Verification items for the finished model (mm, model axes). Face numbers are marked on the shaded views. A direction names the side the tool comes from. Round coordinates to 2 decimals unless told otherwise and drop trailing zeros. Write each loop counter-clockwise with the first axis right and the second up, starting at its lowest first coordinate (ties: lowest second). Pieces come first, ordered by that corner, then holes. Notation, with made-up numbers: (-35, -27) -> (18, -27) arc R24 ccw to (18, -10) -> close; hole circle Ø11 at (83, -1). An arc over 180 degrees is marked (long way). Use CSV: the item, a comma, the result in double quotes.
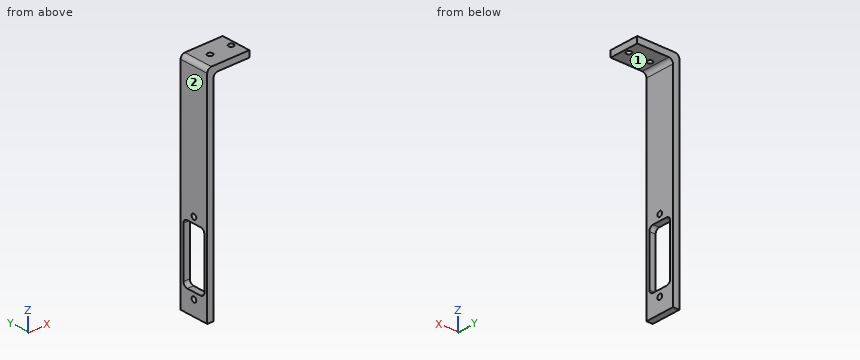
Autodesk Inventor part; units mm, degrees
ref_plane "YZ Plane" through (0, 0, 0) normal (1, 0, 0) x (0, 1, 0)
ref_plane "XZ Plane" through (0, 0, 0) normal (0, 1, 0) x (-1, 0, 0)
ref_plane "XY Plane" through (0, 0, 0) normal (0, 0, 1) x (1, 0, 0)
sketch "Sketch1" plane through (0, 0, 0) normal (0, 1, 0) x (-1, 0, 0)
  line L0 (0, 0) -> (0, -3)
  line L1 (0, -3) -> (15, -3)
  line L2 (17, -5) -> (17, -102.86)
  line L3 (0, 0) -> (18, 0)
  line L4 (20, -2) -> (20, -102.86)
  line L5 (20, -102.86) -> (17, -102.86)
  arc A0 (17, -5) -> (15, -3) centre (15, -5) ccw
  arc A1 (20, -2) -> (18, 0) centre (18, -2) ccw
  point P0 (17, -3)
  point P1 (20, 0)
  dimension "d0" = 3
  dimension "d1" = 17
  dimension "d2" = 99.86
  dimension "d3" = 20
  dimension "d4" = 2
extrude "Extrusion1" add sketch "Sketch1" along normal blind 14
sketch "Sketch2" plane through (0, 0, -3) normal (0, 0, -1) x (-1, 0, 0)
  point P0 (0, 0)
sketch "Sketch3" plane through (0, 0, -3) normal (0, 0, -1) x (-1, 0, 0)
  circle A0 centre (2.3646, 7) radius 1.5
  circle A1 centre (12.3646, 7) radius 1.5
  line L0 (0, 14) -> (15, 14)
  line L1 (0, 0) -> (15, 0)
  dimension "d7" = 3
  dimension "d8" = 3
  dimension "d9" = 14
  dimension "d10" = 7
  dimension "d11" = 10
hole "Hole1" at (-2.3646, 7, -3) at (-12.3646, 7, -3) direction (0, 0, 1) diameter 2.459 depth 8.8 tip angle 118
sketch "Sketch4" plane through (-20, 0, -102.86) normal (-1, 0, 0) x (0, 0, 1)
  line L0 (12, 12.5) -> (35.5, 12.5)
  line L1 (37.5, 10.5) -> (37.5, 3.5)
  line L2 (35.5, 1.5) -> (12, 1.5)
  line L3 (10, 3.5) -> (10, 10.5)
  line L4 (0, 14) -> (100.86, 14)
  line L5 (0, 0) -> (100.86, 0)
  line L6 (0, 0) -> (0, 14)
  circle A0 centre (7, 7) radius 1.5
  circle A1 centre (40.32, 7) radius 1.5
  arc A2 (12, 12.5) -> (10, 10.5) centre (12, 10.5) ccw
  arc A3 (10, 3.5) -> (12, 1.5) centre (12, 3.5) ccw
  arc A4 (37.5, 10.5) -> (35.5, 12.5) centre (35.5, 10.5) ccw
  arc A5 (35.5, 1.5) -> (37.5, 3.5) centre (35.5, 3.5) ccw
  point P0 (102.86, 0)
  point P1 (10, 12.5)
  point P2 (37.5, 1.5)
  point P3 (37.5, 12.5)
  point P4 (10, 1.5)
  dimension "d19" = 27.5
  dimension "d20" = 11
  dimension "d21" = 14
  dimension "d22" = 1.5
  dimension "d23" = 10
  dimension "d24" = 3
  dimension "d25" = 3
  dimension "d26" = 33.32
  dimension "d29" = 7
  dimension "d39" = 2
hole "Hole2" at (-20, 7, -62.54) at (-20, 7, -95.86) direction (1, 0, 0) diameter 2.459 depth 8.8 tip angle 118
extrude "Extrusion2" cut sketch "Sketch4" against normal blind 14 contours L0 A4 L1 A5 L2 A3 L3 A2
equation "\"d10\" = 0.5 * d9"
equation "\"d22\" = -0.5 * d20 + 0.5 * d21"
properties part number "płytka złącza"
Q1. Section check C-C (x = -4.75). Record the cut outline in (y, z), plus the area to 3 significant figures.
Filled in:
outline,"(0, -3) -> (14, -3) -> (14, 0) -> (0, 0) -> close"
area,"42.0 mm²"
Q2. Go/stop test with flat-tipped pins: P1, Ø8, axis at y = 12.5, z = -65, coming from the +X side; P2, Ø1.5, axis at y = 7, z = -95.86, coming from the +X side; P3, Ø7, axis at x = -4.5, y = 7, coming from the -Z side. Record where each tip stops, or that it passes through.
Filled in:
P1,"x = -17"
P2,"through"
P3,"z = -3"
Q3. Section check B-B (z = -62.54). Record the cut outline in (x, y), plus the area to 3 significant figures.
Filled in:
outline,"(-20, 0) -> (-17, 0) -> (-17, 5.77) -> (-20, 5.77) -> close; (-20, 8.23) -> (-17, 8.23) -> (-17, 14) -> (-20, 14) -> close"
area,"34.6 mm²"
Q4. Access from +Z, -Z, +X, -X, +Y, -Y to the whole of each face (thin tool, end or side, straight path). Record for the marked faces 1 and 2.
Filled in:
face 1,"-Z, +X, +Y, -Y"
face 2,"+Z, -Z, -X, +Y, -Y"
Q5. Material ranges on L1, parallel to Z at x = -18.1, y = 7; L2, parallel to Y at x = -17.95, z = -95.86; L3, parallel to X at y = 7, z = -2.3, recorded low to high.
Filled in:
L1,"-102.86 to -97.09, -94.63 to -92.86, -65.36 to -63.77, -61.31 to 0"
L2,"0 to 5.77, 8.23 to 14"
L3,"-20 to -13.59, -11.14 to -3.59, -1.14 to 0"
Q6. Section check D-D (z = -46.5). Record the cut outline in (x, y).
Filled in:
outline,"(-20, 0) -> (-17, 0) -> (-17, 14) -> (-20, 14) -> close"
Q7. Section check A-A (y = 7). Record the cut outline in (x, z), plus the area to 3 significant figures.
Filled in:
outline,"(-20, -102.86) -> (-17, -102.86) -> (-17, -97.09) -> (-20, -97.09) -> close; (-20, -94.63) -> (-17, -94.63) -> (-17, -92.86) -> (-20, -92.86) -> close; (-20, -65.36) -> (-17, -65.36) -> (-17, -63.77) -> (-20, -63.77) -> close; (-20, -61.31) -> (-17, -61.31) -> (-17, -5) arc R2 cw to (-15, -3) -> (-13.59, -3) -> (-13.59, 0) -> (-18, 0) arc R2 ccw to (-20, -2) -> close; (-11.14, -3) -> (-3.59, -3) -> (-3.59, 0) -> (-11.14, 0) -> close; (-1.14, -3) -> (0, -3) -> (0, 0) -> (-1.14, 0) -> close"
area,"248 mm²"
